Input: part model. Units: mm. Frame: model coordinates. Round coordinates to 2 decimals unless told otherwise and drop trailing zeros. Write each question's results on one line, items separated by ' | '.
from build123d import *

# Parameters (mm, degrees)
CHAMFER1_SIZE = 0.1190625


with BuildPart() as part:
    # Sketch2 → Revolve1 (revolve)
    with BuildSketch(Plane(origin=(0, 0, 0), x_dir=(0, 0, -1), z_dir=(1, 0, 0)), mode=Mode.PRIVATE) as revolve1_sk:
        Polygon((-4.527369904, 3.175), (-5.159375, 3.65125), (-5.159375, 4.1275), (-1.719791667, 4.1275), (-1.719791667, 3.65125), (5.159375, 3.65125), (5.159375, 3.175), align=None)
    revolve(revolve1_sk.sketch.rotate(Axis((0, 0, 5.159375), (0, 0, -1)), 90), axis=Axis((0, 0, 5.159375), (0, 0, -1)))

    # Chamfer1
    chamfer1_edges = [part.edges().sort_by_distance(p)[0] for p in [
        (-4.1275, 0, 1.719791667),
        (-4.1275, 0, 5.159375),
    ]]
    chamfer(chamfer1_edges, length=CHAMFER1_SIZE)


solid = part.part
1. Mould query, pull axis Y, two halves, no side actions, for faces 1 (the flat face through (-0.6, -3.3, -5.159)), 2 (the cylindrical face through (-0.48, -3.62, -1.77)), 3 (the cylindrical face through (-2.52, 1.93, -0.25)). Classes: pulls with the +Y half, pulls with the -Y half, needs draft (parallel to the pull), parting line crosses it, or undercut.
Answer:
face 1: needs draft | face 2: parting line crosses it | face 3: undercut
2. Contact query for a flat-ended pin moving along its axis: pin 1 (3 mm diameter, centred on y = 3, z = -1.5, fed in from -X). Output: stop coordinate, or through.
Answer:
pin 1: x = -3.33
3. Line query: line 1 (Y direction, x = 0, z = 2.75) (1 decimal); line 2 (X direction, y = 0.5, z = 0.5); line 3 (Z direction, x = -1.75, y = 3.25). Output: solid intervals per line, ascending. Write a range as [from, to].
Answer:
line 1: [-4.1, -3.2], [3.2, 4.1] | line 2: [-3.62, -3.14], [3.14, 3.62] | line 3: [1.72, 5.16]
